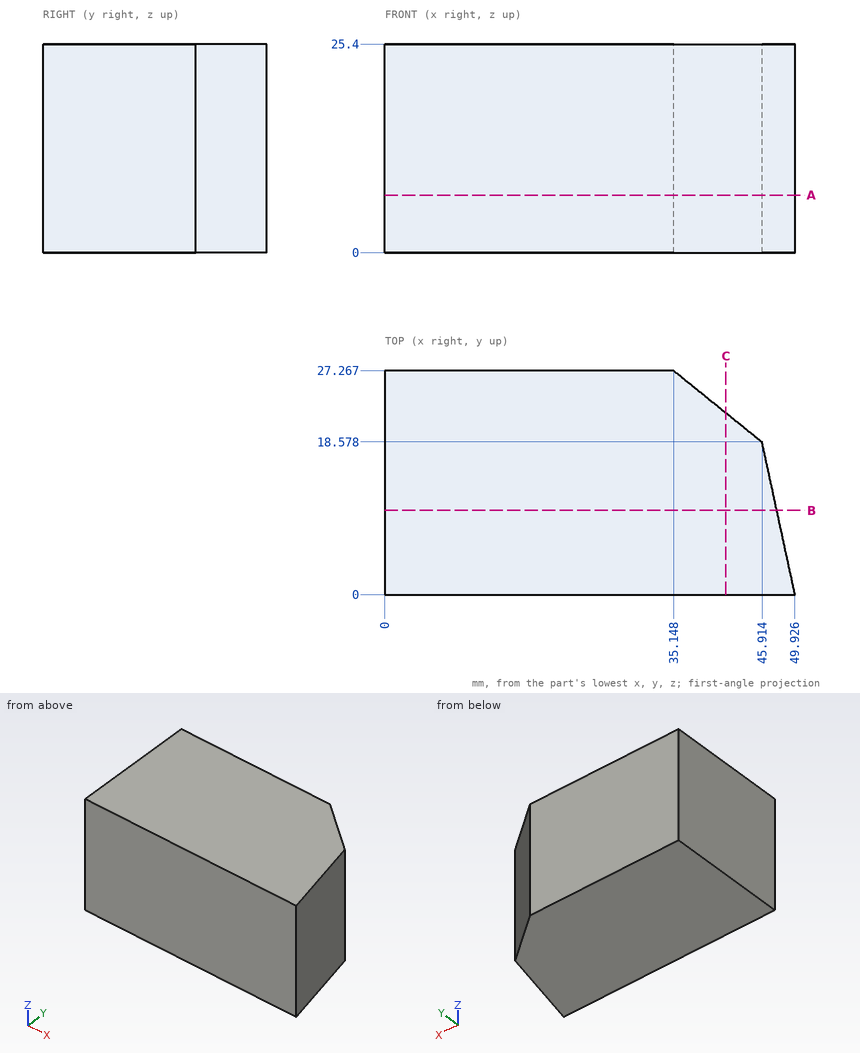
For this review, use the dimensioned drawing (mm, ordinates from the lowest corner) and the shaded views. Coordinates: 2 decimals unless noted, no trailing zeros. Write each loop counter-clockwise with the first axis right and the second up, starting at its lowest first coordinate (ties: lowest second). Pieces come first, ordered by that corner, then holes. Notation, with made-up numbers: (-38, -21.5) - (-25, -21.5) arc R23 cw to (-25, 1.5) - close; hole circle Ø2 at (-8, 83.5). An arc over 180 degrees is marked (long way). Answer as a JSON object with one key per item and string values. Group by question number.
1. Add section C-C (x = 41.5). Give the boundary of the cut face in (y, z).
2. To check wall thickness, follow probe 1 along Y at (x, z) = (38, 8) (1 decimal); probe 2 along X at (y, z) = (15.5, 3.75); probe 3 along X at (y, z) = (14.25, 7). State the ranges of each line that lie inside material, in increasing order.
3. Clearance check with flat-ended pins moving along their axes: pin 1 Ø10 at (y, z) = (22, 10) entering from +X (1 decimal); pin 2 Ø6 at (y, z) = (22, 20) entering from +X. State where each tip first meets the part, or that it passes through.
4. Add section B-B (y = 10.25). Give the boundary of the cut face in (x, z), plus the area to 3 significant figures.
5. Add section A-A (z = 7). Give the boundary of the cut face in (x, y) (1 decimal), plus the area to 3 significant figures.
Findings:
{
 "1": {"outline": "(0, 0) - (22.14, 0) - (22.14, 25.4) - (0, 25.4) - close"},
 "2": {"probe 1": "0 to 25", "probe 2": "0 to 46.58", "probe 3": "0 to 46.85"},
 "3": {"pin 1": "x = 46.3", "pin 2": "x = 45.39"},
 "4": {"outline": "(0, 0) - (47.71, 0) - (47.71, 25.4) - (0, 25.4) - close", "area": "1,210 mm²"},
 "5": {"outline": "(0, 0) - (49.9, 0) - (45.9, 18.6) - (35.1, 27.3) - (0, 27.3) - close", "area": "1,240 mm²"}
}
